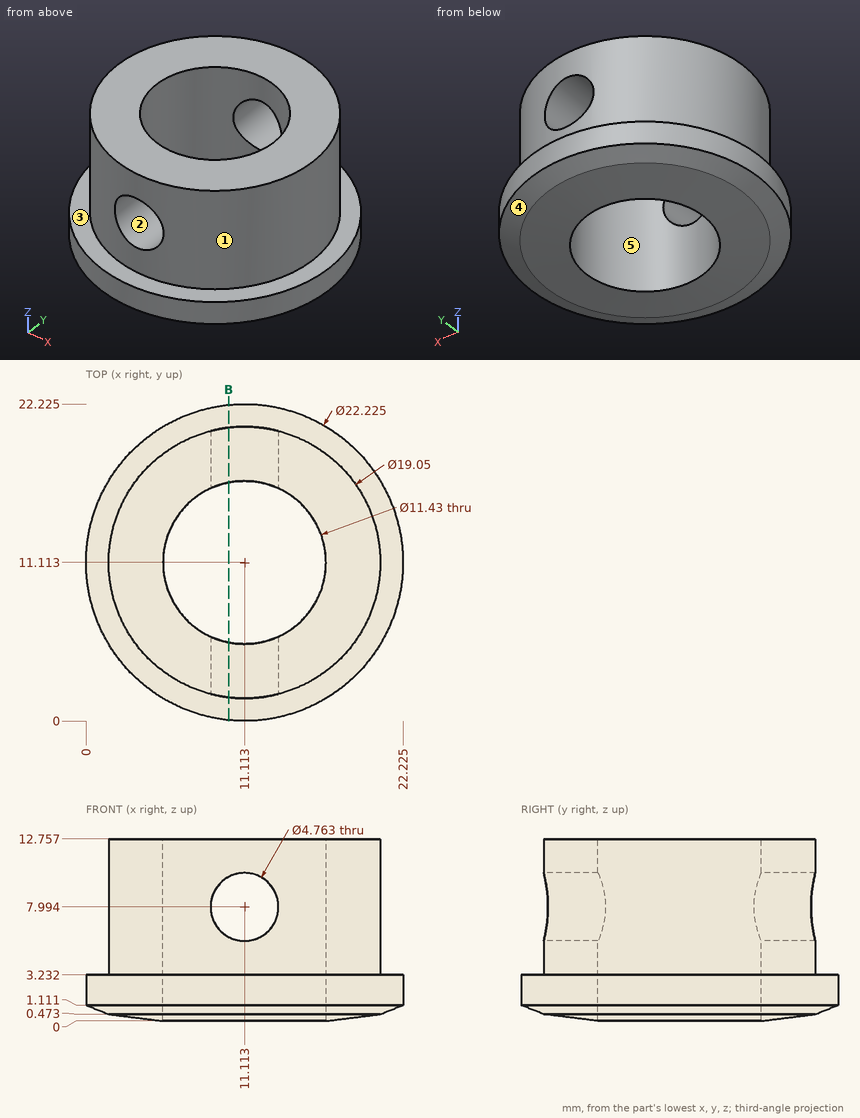
For this review, use the dimensioned drawing (mm, ordinates from the lowest corner) and the shaded views. A direction names the side the tool comes from. Round coordinates to 2 decimals unless told otherwise and drop trailing zeros. Answer as a JSON object with one key per item and string values.
1. For pin 1 Ø6 at (y, z) = (7, 11) entering from +X; pin 2 Ø3 at (x, z) = (19, 9) entering from +Y; pin 3 Ø6 at (y, z) = (6, 5) entering from -X; pin 4 Ø4.5 at (x, z) = (11.11, 7.99) entering from +Y, all flat-tipped, find the tip position at first contact; note any pin that passes through.
Response values:
{"pin 1": "stops at x = 20.57", "pin 2": "stops at y = 18.18", "pin 3": "stops at x = 0.33", "pin 4": "passes through"}
2. Draft analysis for pull direction Y (two halves, no side actions). For the marked faces 3, 4 and 5, state which applies: +Y half, -Y half, draft (parallel to the pull), parting line (faces both ways), or undercut.
Response values:
{"face 3": "draft", "face 4": "parting line", "face 5": "undercut"}
3. We need section B-B on x = 10. Count the separate pieces of the cut face and the enclosed holes in it.
Response values:
{"separate pieces": "4", "enclosed holes": "0"}
4. To check wall thickness, follow line 1 along Y through (x, z) = (14.25, 4.5) (1 decimal); line 2 along Y through (x, z) = (11.5, 11.25) (1 decimal); line 3 along X through (y, z) = (6.5, 5.75) (1 decimal). State the ranges of each line that lie inside material, in increasing order.
Response values:
{"line 1": "y = 2.1 to 6.3, 15.9 to 20.1", "line 2": "y = 1.6 to 5.4, 16.8 to 20.6", "line 3": "x = 2.8 to 7.7, 14.5 to 19.4"}
5. Tool access review of the marked faces 1 and 2: name each direction out of +Z, -Z, +X, -X, +Y, -Y from which nothing blocks a thin tool from reaching the whole face with its end or side.
Response values:
{"face 1": "+Z", "face 2": "+Y, -Y"}
